Verification items for the finished model (mm, model axes). Coordinates: 2 decimals unless noted, no trailing zeros. Order: outer loops, then holes, each group sorted by start corner. A loop starts at its lowest first (then second) coordinate and runs counter-clockwise, first axis right, second up. Notation, with made-up numbers: (67.5, 58) -> (112.5, 58) arc R30 ccw to (112.5, 87) -> close; hole circle Ø4 at (36, 2). An arc over 180 degrees is marked (long way). Answer as CSV lines item,"result".
```python
from build123d import *

# Parameters (mm, degrees)
SKETCH1_R           = 5
BOSS_EXTRUDE1_DEPTH = 5


with BuildPart() as part:
    # Sketch1 → Boss-Extrude1 (new body)
    with BuildSketch(Plane(origin=(0, 0, 0), x_dir=(1, 0, 0), z_dir=(0, 1, 0))):
        with BuildLine():
            Line((0, -10), (0, 10))
            Line((0, 10), (20, 10))
            ThreePointArc((20, 10), (30, 0), (20, -10))
            Line((20, -10), (0, -10))
        make_face()
        with Locations(Location((20, 0, 0), (0, 0, 270))):
            Circle(SKETCH1_R, mode=Mode.SUBTRACT)
    extrude(amount=BOSS_EXTRUDE1_DEPTH)


solid = part.part
```
Item 1: Depth check by flat-ended pin: pin 1 Ø6 at (x, z) = (20, 0) entering from -Y. Enter the tip coordinate at first touch or a pass-through.
Answer list:
pin 1,"through"
Item 2: Thickness scan on line 1 (X direction, y = 2.1, z = 0); line 2 (X direction, y = 2.3, z = -1.5); line 3 (Z direction, x = 17.5, y = 4.65). Record the ranges inside material, lowest first.
Answer list:
line 1,"0 to 15, 25 to 30"
line 2,"0 to 15.23, 24.77 to 29.89"
line 3,"-10 to -4.33, 4.33 to 10"
Item 3: Section check A-A, the plane z = 0. Record the boundary of the cut face in (x, y).
Answer list:
outline,"(0, 0) -> (15, 0) -> (15, 5) -> (0, 5) -> close; (25, 0) -> (30, 0) -> (30, 5) -> (25, 5) -> close"
Item 4: Section check C-C, the plane y = 3.25. Record the boundary of the cut face in (x, z), plus the area to 3 significant figures.
Answer list:
outline,"(0, -10) -> (20, -10) arc R10 ccw to (20, 10) -> (0, 10) -> close; hole circle Ø10 at (20, 0)"
area,"479 mm2"
Item 5: Section check D-D, the plane z = 6.5. Record the boundary of the cut face in (x, y).
Answer list:
outline,"(0, 0) -> (27.6, 0) -> (27.6, 5) -> (0, 5) -> close"
Item 6: Release check for a two-part mould opening along X. For faces 1 (the flat face through (12, 5, 0)), 2 (the flat face through (0, 2, 0)), 3 (the cylindrical face through (15.12, 2.46, -1.08)) record: +X half, -X half, draft (parallel to the pull), parting line (faces both ways), or undercut.
Answer list:
face 1,"draft"
face 2,"-X half"
face 3,"undercut"
Item 7: Section check B-B, the plane x = 24. Record the boundary of the cut face in (y, z), plus the area to 3 significant figures.
Answer list:
outline,"(0, -9.17) -> (5, -9.17) -> (5, -3) -> (0, -3) -> close; (0, 3) -> (5, 3) -> (5, 9.17) -> (0, 9.17) -> close"
area,"61.7 mm2"
